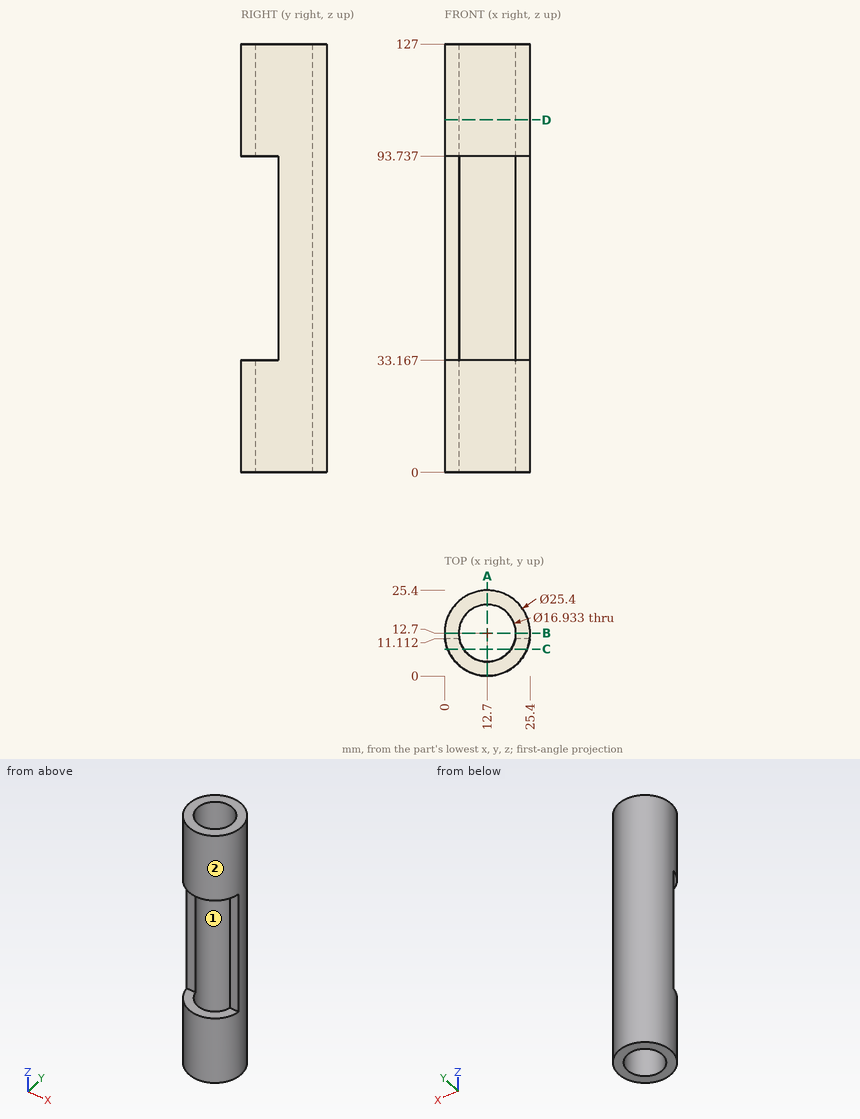
Verification items for this drawing (mm, ordinates from the low corner). Give positions to 0.01 mm unless a question says otherwise; leave off trailing zeros. Order: outer loops, then holes, each group sorted by start corner. A loop starts at its lowest first (then second) coordinate and runs counter-clockwise, first axis right, second up.
1) Material ranges on probe 1 along Z at (x, y) = (12.75, 2.75); probe 2 along Y at (x, z) = (12.7, 58.5); probe 3 along Y at (x, z) = (12.7, 31), recorded low to high.
Results are:
probe 1: z = 0 to 33.17, 93.74 to 127
probe 2: y = 21.17 to 25.4
probe 3: y = 0 to 4.23, 21.17 to 25.4
2) Draft check along X on the marked faces 1 and 2. Enter one of: released by +X, released by -X, zero draft, split by the parting line, or undercut.
Results are:
face 1: undercut
face 2: split by the parting line
3) Cross-section at D-D (z = 104.5). Record the boundary of the cut face in (x, y).
Results are:
outline: circle Ø25.4 at (12.7, 12.7); hole circle Ø16.93 at (12.7, 12.7)
4) Gauge pin test, flat ends, axial feed: pin 1 (3 mm diameter, centred on y = 18, z = 100, fed in from +X); pin 2 (10 mm diameter, centred on x = 13, z = 88, fed in from -Y); pin 3 (6 mm diameter, centred on x = 14.5, z = 77, fed in from -Y) (1 decimal); pin 4 (10 mm diameter, centred on x = 9, y = 5.5, fed in from +Z). Record the tip position at first contact, or that the pin passes through.
Results are:
pin 1: stops at x = 24.82
pin 2: stops at y = 19.3
pin 3: stops at y = 19.7
pin 4: stops at z = 127
5) Cross-section at B-B (y = 12.7). Record the boundary of the cut face in (x, z).
Results are:
outline: (0, 0) - (4.23, 0) - (4.23, 127) - (0, 127) - close; (21.17, 0) - (25.4, 0) - (25.4, 127) - (21.17, 127) - close
6) Cross-section at C-C (y = 8). Record the boundary of the cut face in (x, z), then the cut area to 3 significant figures.
Results are:
outline: (0.9, 0) - (5.66, 0) - (5.66, 33.17) - (0.9, 33.17) - close; (0.9, 93.74) - (5.66, 93.74) - (5.66, 127) - (0.9, 127) - close; (19.74, 0) - (24.5, 0) - (24.5, 33.17) - (19.74, 33.17) - close; (19.74, 93.74) - (24.5, 93.74) - (24.5, 127) - (19.74, 127) - close
area: 632 mm2
7) Cross-section at A-A (x = 12.7). Record the boundary of the cut face in (y, z).
Results are:
outline: (0, 0) - (4.23, 0) - (4.23, 33.17) - (0, 33.17) - close; (0, 93.74) - (4.23, 93.74) - (4.23, 127) - (0, 127) - close; (21.17, 0) - (25.4, 0) - (25.4, 127) - (21.17, 127) - close
